Here's the drawing with two shaded views (mm, measured from the low corner). I have some questions. Give positions to 0.01 mm unless a question says otherwise; leave off trailing zeros. Write each loop counter-clockwise with the first axis right and the second up, starting at its lowest first coordinate (ties: lowest second). Pieces come first, ordered by that corner, then holes. Notation, with made-up numbers: M 58.5,-1.5 L 106.5,-1.5 A20 cw 106.5,5.5 Z; hole C 77,-5.75 d10. An arc over 180 degrees is marked long. Use one line per item in the form item = value. Start each with the question number.
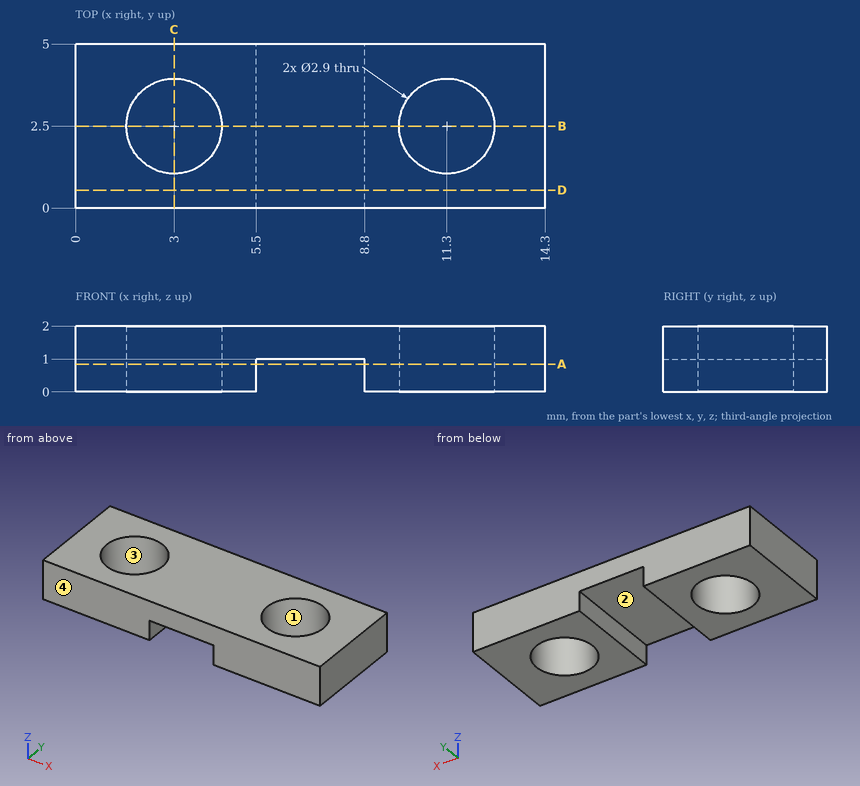
1) Suppose I cut it at C-C, the plane x = 3. List the corners of the cut face in (y, z) for me, and give its area (3 significant figures).
2) Suppose I cut it at D-D, the plane y = 0.55. List the corners of the cut face in (x, z) for me, and give its area (3 significant figures).
3) Thinking about a two-plate mould opening in Y: for the marked faces 1, 2, 3 and 4, which applies, released by +Y, released by -Y, zero draft, split by the parting line, or undercut?
4) Please list where these lines run through material, in increasing order: line 1 (Y direction, x = 3, z = 1.5); line 2 (X direction, y = 1.3, z = 0.6); line 3 (X direction, y = 2, z = 1.35).
5) Suppose I cut it at A-A, the plane z = 0.85. List the corners of the cut face in (x, y) for me.
6) Will these pins go through, and if not, where does the flat tip stop? P1, Ø1, axis at x = 7, y = 1.5, coming from the -Z side; P2, Ø1.7, axis at x = 3, y = 2.5, coming from the +Z side; P3, Ø1.1, axis at y = 3.5, z = 0.5, coming from the -X side.
7) Suppose I cut it at B-B, the plane y = 2.5. List the corners of the cut face in (x, z) for me, and give its area (3 significant figures).
Checks:
q1.outline = M 0,0 L 1.05,0 L 1.05,2 L 0,2 Z; M 3.95,0 L 5,0 L 5,2 L 3.95,2 Z
q1.area = 4.20 mm^2
q2.outline = M 0,0 L 5.5,0 L 5.5,1 L 8.8,1 L 8.8,0 L 14.3,0 L 14.3,2 L 0,2 Z
q2.area = 25.3 mm^2
q3.face_1 = undercut
q3.face_2 = zero draft
q3.face_3 = undercut
q3.face_4 = released by -Y
q4.line_1 = 0 to 1.05, 3.95 to 5
q4.line_2 = 0 to 2.19, 3.81 to 5.5, 8.8 to 10.49, 12.11 to 14.3
q4.line_3 = 0 to 1.64, 4.36 to 9.94, 12.66 to 14.3
q5.outline = M 0,0 L 5.5,0 L 5.5,5 L 0,5 Z; M 8.8,0 L 14.3,0 L 14.3,5 L 8.8,5 Z; hole C 3,2.5 d2.9; hole C 11.3,2.5 d2.9
q6.P1 = 1
q6.P2 = through
q6.P3 = 0
q7.outline = M 0,0 L 1.55,0 L 1.55,2 L 0,2 Z; M 4.45,0 L 5.5,0 L 5.5,1 L 8.8,1 L 8.8,0 L 9.85,0 L 9.85,2 L 4.45,2 Z; M 12.75,0 L 14.3,0 L 14.3,2 L 12.75,2 Z
q7.area = 13.7 mm^2
